```python
from build123d import *

# Parameters (mm, degrees)
SKETCH1_W                               = 74.5
SKETCH1_H                               = 104.5
SKETCH1_W_2                             = 70.5
SKETCH1_H_2                             = 100.5
BOSS_EXTRUDE1_ABOVE_BOARD_SURFACE_DEPTH = 5
SKETCH2_W                               = 104.5
SKETCH2_H                               = 74.5
BOSS_EXTRUDE2_UNDER_23MM_DEPTH          = 23
SKETCH3_W                               = 104.5
SKETCH3_H                               = 74.5
BOSS_EXTRUDE3_BOTTOM_COVER_2MM_DEPTH    = 2
SKETCH4_W                               = 5
SKETCH4_H                               = 3.5
BOSS_EXTRUDE4_ANCHOR_PINS_DEPTH         = 2
SKETCH5_W                               = 150
SKETCH5_H                               = 45
CUT_EXTRUDE1_CUT_USB_DEPTH              = 20
CUT_EXTRUDE1_CUT_USB_DRAFT              = -20
FILLET1_R                               = 2
CHAMFER2_SIZE                           = 1.5
SKETCH6_W                               = 10
SKETCH6_H                               = 3
BOSS_EXTRUDE1_DEPTH                     = 10
SKETCH7_W                               = 53
SKETCH7_H                               = 15
CUT_EXTRUDE1_DEPTH                      = 10


with BuildPart() as part:
    # Sketch1 → Boss-Extrude1-above-board-surface (new body)
    with BuildSketch(Plane(origin=(0, 0, 0), x_dir=(0, 1, 0), z_dir=(0, 0, 1))):
        Rectangle(SKETCH1_W, SKETCH1_H)
        Rectangle(SKETCH1_W_2, SKETCH1_H_2, mode=Mode.SUBTRACT)
    extrude(amount=BOSS_EXTRUDE1_ABOVE_BOARD_SURFACE_DEPTH)

    # Sketch2 → Boss-Extrude2-under-23mm (add)
    with BuildSketch(Plane(origin=(0, 0, 0), x_dir=(1, 0, 0), z_dir=(0, 0, -1))):
        Rectangle(SKETCH2_W, SKETCH2_H)
        Polygon((-50.25, 32.25), (-40.25, 32.25), (-40.25, 35.25), (50.25, 35.25), (50.25, -35.25), (-40.25, -35.25), (-40.25, -32.25), (-50.25, -32.25), align=None, mode=Mode.SUBTRACT)
    extrude(amount=BOSS_EXTRUDE2_UNDER_23MM_DEPTH)

    # Sketch3 → Boss-Extrude3-bottom-cover-2mm (add)
    with BuildSketch(Plane(origin=(0, 0, -23), x_dir=(1, 0, 0), z_dir=(0, 0, -1))):
        Rectangle(SKETCH3_W, SKETCH3_H)
    extrude(amount=BOSS_EXTRUDE3_BOTTOM_COVER_2MM_DEPTH)

    # Sketch4 → Boss-Extrude4-anchor-pins (add)
    with BuildSketch(Plane.XY.offset(2.1)):
        with Locations((-22.75, 35.5)):
            Rectangle(SKETCH4_W, SKETCH4_H)
        with Locations((22.75, 35.5)):
            Rectangle(SKETCH4_W, SKETCH4_H)
        with Locations((0, -35.5)):
            Rectangle(SKETCH4_W, SKETCH4_H)
    extrude(amount=BOSS_EXTRUDE4_ANCHOR_PINS_DEPTH)


with BuildPart() as cut_extrude1_cut_usb_tool:
    # Sketch5 → Cut-Extrude1-cut-usb (with draft: the straight prism first)
    with BuildSketch(Plane.XY.offset(5)):
        Rectangle(SKETCH5_W, SKETCH5_H)
    extrude(amount=-CUT_EXTRUDE1_CUT_USB_DEPTH)
    # Cut-Extrude1-cut-usb: the draft: its side faces are tilted about the plane it starts from
    cut_extrude1_cut_usb_sides = [cut_extrude1_cut_usb_tool.faces().sort_by_distance(p)[0] for p in [
        (0, -22.5, -5),
        (75, 0, -5),
        (0, 22.5, -5),
        (-75, 0, -5),
    ]]
    draft(cut_extrude1_cut_usb_sides, Plane.XY.offset(5), CUT_EXTRUDE1_CUT_USB_DRAFT)


with BuildPart() as part_1:
    add(part.part)

    # Cut-Extrude1-cut-usb: cut by cut_extrude1_cut_usb_tool
    add(cut_extrude1_cut_usb_tool.part, mode=Mode.SUBTRACT)

    # Fillet1
    fillet1_edges = [part_1.edges().sort_by_distance(p)[0] for p in [
        (52.25, -37.25, -10),
        (-52.25, -37.25, -10),
        (-52.25, 37.25, -10),
        (52.25, 37.25, -10),
    ]]
    fillet(fillet1_edges, radius=FILLET1_R)

    # Chamfer2
    chamfer2_edges = [part_1.edges().sort_by_distance(p)[0] for p in [
        (20.25, 35.25, 3.1),
        (25.25, 35.25, 3.1),
        (-25.25, 35.25, 3.1),
        (-20.25, 35.25, 3.1),
        (2.5, -35.25, 3.1),
        (-2.5, -35.25, 3.1),
    ]]
    chamfer(chamfer2_edges, length=CHAMFER2_SIZE - 0.0001)  # a hair under: the kernel refuses the full size

    # Sketch6 → Boss-Extrude1 (add)
    with BuildSketch(Plane.XY.offset(-13)):
        with Locations((35.25, -33.75)):
            Rectangle(SKETCH6_W, SKETCH6_H)
        with Locations((35.25, 33.75)):
            Rectangle(SKETCH6_W, SKETCH6_H)
    extrude(amount=-BOSS_EXTRUDE1_DEPTH)

    # Sketch7 → Cut-Extrude1 (cut)
    with BuildSketch(Plane.XY.offset(-23)):
        with Locations((-4.75, 27.25)):
            Rectangle(SKETCH7_W, SKETCH7_H)
        with Locations((-4.75, -27.25)):
            Rectangle(SKETCH7_W, SKETCH7_H)
    extrude(amount=-CUT_EXTRUDE1_DEPTH, mode=Mode.SUBTRACT)


solid = part_1.part
```
Geometry: final body of the model. Coordinates: model frame, mm. A direction names the side the tool comes from. Coordinates: 2 decimals unless noted, no trailing zeros. Order: outer loops, then holes, each group sorted by start corner. A loop starts at its lowest first (then second) coordinate and runs counter-clockwise, first axis right, second up. Notation, with made-up numbers: (83, 74) - (98, 74) arc R22 ccw to (98, 98) - close; hole circle Ø3 at (-6.5, 68.25). An arc over 180 degrees is marked (long way). Write each question's results on one line, items separated by ' | '.
(1) Mould query, pull axis Y, two halves, no side actions, for faces 1 (the face through (-51.26, -18.91, -4.86)), 2 (the face through (-51.68, 36.65, -10.21)), 3 (the face through (-8, 36, 5)). Classes: +Y half, -Y half, draft (parallel to the pull), parting line (faces both ways), or undercut.
Values found:
face 1: undercut | face 2: +Y half | face 3: draft
(2) Line query: line 1 (Y direction, x = -48, z = -18); line 2 (X direction, y = -10.5, z = -17); line 3 (Y direction, x = -13.5, z = -22.5). Output: solid intervals per line, ascending. Write a range as [from, to].
Values found:
line 1: y = [-37.25, -32.25], [32.25, 37.25] | line 2: x = [-52.25, -50.25], [50.25, 52.25] | line 3: y = [-37.25, -35.25], [35.25, 37.25]
(3) Set-up query: faces 4 (the face through (-31.25, 27, -24)), 5 (the face through (40.25, -34, -18)), 6 (the face through (-1, -37.25, -10)), 7 (the face through (-51.26, 18.91, -4.86)). Return all of +Z, -Z, +X, -X, +Y, -Y with unobstructed straight access to the full face (end or side cutting, diameter ignored); none if empty.
Values found:
face 4: +Z, -Z | face 5: +Z | face 6: +Z, -Z, +X, -X, -Y | face 7: +Z, +X, -X
(4) Section query B-B, the plane y = 31. Return the cut outline in (x, z), plus the area to 3 significant figures.
Values found:
outline: (-52.25, -25) - (-31.25, -25) - (-31.25, -23) - (-50.25, -23) - (-50.25, 5) - (-52.25, 5) - close; (21.75, -25) - (52.25, -25) - (52.25, 5) - (50.25, 5) - (50.25, -23) - (21.75, -23) - close | area: 215 mm²
(5) Section query D-D, the plane x = -37. Return the cut outline in (y, z), plus the area to 3 significant figures.
Values found:
outline: (-37.25, -25) - (37.25, -25) - (37.25, 5) - (35.25, 5) - (35.25, -23) - (-35.25, -23) - (-35.25, 5) - (-37.25, 5) - close | area: 261 mm²
(6) Section query A-A, the plane x = -22. Return the cut outline in (y, z).
Values found:
outline: (-37.25, -25) - (-34.75, -25) - (-34.75, -23) - (-35.25, -23) - (-35.25, 5) - (-37.25, 5) - close; (-19.75, -25) - (19.75, -25) - (19.75, -23) - (-19.75, -23) - close; (33.75, 2.1) - (35.25, 2.1) - (35.25, -23) - (34.75, -23) - (34.75, -25) - (37.25, -25) - (37.25, 5) - (35.25, 5) - (35.25, 4.1) - (33.75, 4.1) - close
(7) Section query C-C, the plane z = -8. Return the cut outline in (x, y).
Values found:
outline: (-52.25, -35.25) arc R2 ccw to (-50.25, -37.25) - (50.25, -37.25) arc R2 ccw to (52.25, -35.25) - (52.25, -17.77) - (50.25, -17.77) - (50.25, -35.25) - (-40.25, -35.25) - (-40.25, -32.25) - (-50.25, -32.25) - (-50.25, -17.77) - (-52.25, -17.77) - close; (-52.25, 17.77) - (-50.25, 17.77) - (-50.25, 32.25) - (-40.25, 32.25) - (-40.25, 35.25) - (50.25, 35.25) - (50.25, 17.77) - (52.25, 17.77) - (52.25, 35.25) arc R2 ccw to (50.25, 37.25) - (-50.25, 37.25) arc R2 ccw to (-52.25, 35.25) - close
(8) First-contact query: pin 1 Ø6 at (x, y) = (-35, -26.5) entering from +Z; pin 2 Ø1 at (x, y) = (-51.5, -4.5) entering from +Z. Flat tips, straight axial feed; report the tip coordinate or a pass-through.
Values found:
pin 1: stops at z = -23 | pin 2: stops at z = -15
